Design review of the part built by this model. Coordinates are the model's own, in mm. Coordinates: 2 decimals unless noted, no trailing zeros. Order: outer loops, then holes, each group sorted by start corner. A loop starts at its lowest first (then second) coordinate and runs counter-clockwise, first axis right, second up. Notation, with made-up numbers: (-29.5, 69) - (3.5, 69) arc R32 cw to (3.5, 108) - close; hole circle Ø11 at (2, 7.25). An arc over 180 degrees is marked (long way). Write item = value, one per line. Start each with the question number.
```python
from build123d import *

# Parameters (mm, degrees)
SKETCH1_R                        = 9.525
BOSS_EXTRUDE1_DEPTH              = 342.9
SKETCH2_R                        = 6.35
BOSS_EXTRUDE2_DEPTH              = 9.779
F_12_24_TAPPED_HOLE1_D           = 4.4958
F_12_24_TAPPED_HOLE1_DEPTH       = 25.4
F_12_24_TAPPED_HOLE1_CSINK_D     = 6.35
F_12_24_TAPPED_HOLE1_CSINK_ANGLE = 82
F_12_24_TAPPED_HOLE1_TIP         = 1.350674586
BOSS_EXTRUDE3_START              = 9.779
SKETCH5_R                        = 6.35
BOSS_EXTRUDE3_DEPTH              = 9.779
F_12_24_TAPPED_HOLE2_D           = 4.4958
F_12_24_TAPPED_HOLE2_DEPTH       = 25.4
F_12_24_TAPPED_HOLE2_CSINK_D     = 6.35
F_12_24_TAPPED_HOLE2_CSINK_ANGLE = 82
F_12_24_TAPPED_HOLE2_TIP         = 1.350674586


with BuildPart() as part:
    # Sketch1 → Boss-Extrude1 (new body)
    with BuildSketch(Plane.XY):
        Circle(SKETCH1_R)
    extrude(amount=BOSS_EXTRUDE1_DEPTH)

    # Sketch2 → Boss-Extrude2 (add)
    with BuildSketch(Plane.XY.offset(342.9)):
        Circle(SKETCH2_R)
    extrude(amount=BOSS_EXTRUDE2_DEPTH)

    # #12-24 Tapped Hole1
    with Locations(Plane.XY.offset(352.679)):
        with Locations((0, 0)):
            CounterSinkHole(F_12_24_TAPPED_HOLE1_D / 2, F_12_24_TAPPED_HOLE1_CSINK_D / 2, depth=F_12_24_TAPPED_HOLE1_DEPTH, counter_sink_angle=F_12_24_TAPPED_HOLE1_CSINK_ANGLE)
            with Locations((0, 0, -(F_12_24_TAPPED_HOLE1_DEPTH + F_12_24_TAPPED_HOLE1_TIP / 2))):  # 118° drill point
                Cone(0, F_12_24_TAPPED_HOLE1_D / 2, F_12_24_TAPPED_HOLE1_TIP, mode=Mode.SUBTRACT)

    # Sketch5 → Boss-Extrude3 (add)
    with BuildSketch(Plane(origin=(0, 0, 0), x_dir=(-1, 0, 0), z_dir=(0, 0, -1)).offset(BOSS_EXTRUDE3_START)):
        with Locations(Location((0, 0, 0), (0, 0, 180))):
            Circle(SKETCH5_R)
    extrude(amount=-BOSS_EXTRUDE3_DEPTH)

    # #12-24 Tapped Hole2
    with Locations(Plane(origin=(0, 0, -9.779), x_dir=(-1, 0, 0), z_dir=(0, 0, -1))):
        with Locations((0, 0)):
            CounterSinkHole(F_12_24_TAPPED_HOLE2_D / 2, F_12_24_TAPPED_HOLE2_CSINK_D / 2, depth=F_12_24_TAPPED_HOLE2_DEPTH, counter_sink_angle=F_12_24_TAPPED_HOLE2_CSINK_ANGLE)
            with Locations((0, 0, -(F_12_24_TAPPED_HOLE2_DEPTH + F_12_24_TAPPED_HOLE2_TIP / 2))):  # 118° drill point
                Cone(0, F_12_24_TAPPED_HOLE2_D / 2, F_12_24_TAPPED_HOLE2_TIP, mode=Mode.SUBTRACT)


solid = part.part
```
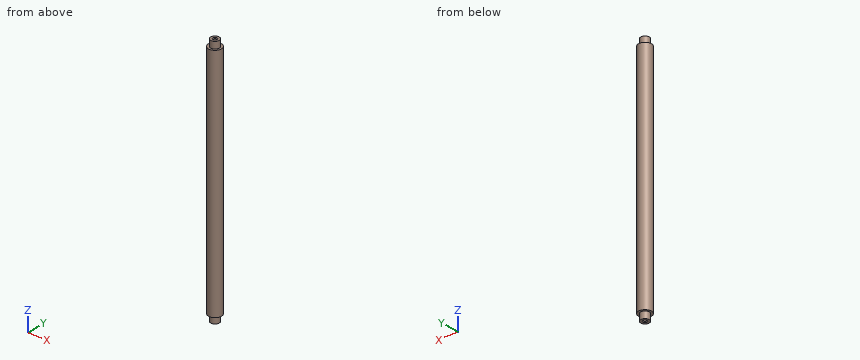
Item 1: For line 1 (Y direction, x = 0, z = 0.75) (3 decimals); line 2 (Z direction, x = 8.5, y = -1); line 3 (Y direction, x = 0.5, z = 316.5), list the stretches that pass through material, from the lowest coordinate up.
Item 2: Add section A-A on z = 231.5. Give the boundary of the cut face in (x, y) (3 decimals), plus the area to 3 significant figures.
Item 3: For P1, Ø1.5, axis at y = -4, z = 44, coming from the -X side; P2, Ø2, axis at y = -5.5, z = 142.5, coming from the -X side (3 decimals); P3, Ø1.5, axis at x = -7.5, y = -6.5, coming from the +Z side, all flat-tipped, find the tip position at first contact; note any pin that passes through.
Worked out:
q1.line_1 = -9.525 to -2.248, 2.248 to 9.525
q1.line_2 = 0 to 342.9
q1.line_3 = -9.51 to 9.51
q2.outline = circle Ø19.05 at (0, 0)
q2.area = 285 mm2
q3.P1 = -8.95
q3.P2 = -8.395
q3.P3 = 342.9
